Autodesk Inventor part; units mm, degrees
ref_plane "Work Plane1" through (0, 0, 6.25) normal (0, 0, 1) x (1, 0, 0)
ref_plane "YZ Plane" through (0, 0, 0) normal (1, 0, 0) x (0, 1, 0)
ref_plane "XZ Plane" through (0, 0, 0) normal (0, 1, 0) x (-1, 0, 0)
sketch "Sketch1" plane through (0, 0, 0) normal (0, 1, 0) x (-1, 0, 0)
  line L0 (0, -8.8201) -> (0, 9.1707)
  line L1 (0, -6.25) -> (0, 6.25)
  line L2 (0, -6.25) -> (1.5, -6.25)
  line L3 (1.5, -6.25) -> (1.5, 3.75)
  line L4 (1.5, 3.75) -> (2.75, 3.75)
  line L5 (2.75, 3.75) -> (2.75, 4.75)
  arc A0 (2.75, 4.75) -> (0, 6.25) centre (0, 2.9792) ccw
  line L6 (3.5295, 0) -> (-0.5882, 0)
  point P0 (0, 0)
  dimension "d0" = 10
  dimension "d1" = 3
  dimension "d2" = 2.5
  dimension "d3" = 5.5
  dimension "d4" = 1
revolve "Revolution1" add sketch "Sketch1" angle 360 about axis through (0, 0, -10) along (0, 0, 1)
ref_plane "Work Plane1" through (0, 0, 6.25) normal (0, 0, 1) x (1, 0, 0)
sketch "Sketch2" plane through (0, 0, 6.25) normal (0, 0, 1) x (1, 0, 0)
  line L0 (-1.35, -0.35) -> (1.35, -0.35)
  line L1 (1.35, -0.35) -> (1.35, 0.35)
  line L2 (1.35, 0.35) -> (-1.35, 0.35)
  line L3 (-1.35, 0.35) -> (-1.35, -0.35)
  line L4 (-1.35, -0.35) -> (1.35, 0.35) construction
  line L5 (1.35, -0.35) -> (-1.35, 0.35) construction
  line L6 (0.35, -1.35) -> (-0.35, -1.35)
  line L7 (-0.35, -1.35) -> (-0.35, 1.35)
  line L8 (-0.35, 1.35) -> (0.35, 1.35)
  line L9 (0.35, 1.35) -> (0.35, -1.35)
  line L10 (0.35, -1.35) -> (-0.35, 1.35) construction
  line L11 (-0.35, -1.35) -> (0.35, 1.35) construction
  point P0 (0, 0)
  dimension "d6" = 2.7
  dimension "d7" = 0.7
extrude "Extrusion1" cut sketch "Sketch2" against normal blind 1
thread "Thread1"
properties part number "empty"
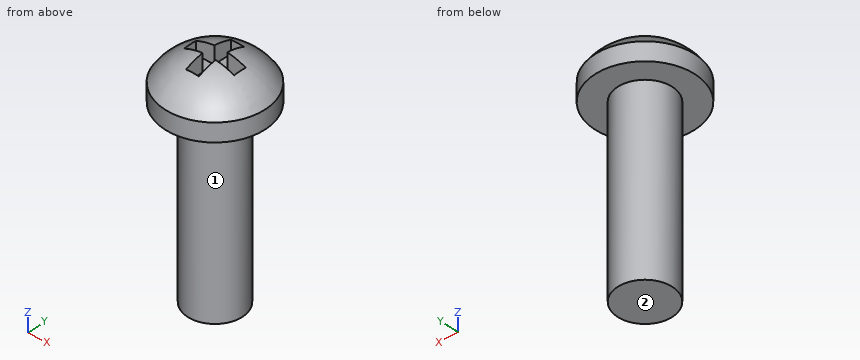
Design review of the part built by this model. Coordinates are the model's own, in mm. Face numbers are marked on the shaded views. A direction names the side the tool comes from. Round coordinates to 2 decimals unless told otherwise and drop trailing zeros. Loops run counter-clockwise (first coordinate to the right, second up) from the corner with the lowest first, then second, coordinate; pieces in that order, holes last. Notation, with made-up numbers: (16.5, -14.75) - (41.5, -14.75) arc R24 ccw to (41.5, 6.25) - close; hole circle Ø5 at (59, -35.5). An arc over 180 degrees is marked (long way). One line per item, written item: value. Start each with the question number.
1) Consider section A-A on z = -1.75. Give the boundary of the cut face in (x, y).
2) Consider section B-B on z = 4.5. Give the boundary of the cut face in (x, y), then the cut area to 3 significant figures.
3) Insertion check: pin 1 Ø3 at (x, y) = (-2, 1) entering from +Z; pin 2 Ø1.1 at (x, z) = (1, 5.5) entering from -Y; pin 3 Ø0.6 at (x, z) = (0, 5.5) entering from +Y. Each pin has a flat end and moves straight along its axis. Give the tip position at first contact, or say it passes through.
4) For the marked faces 1 and 2, list the 3-axis set-ups (+Z, -Z, +X, -X, +Y, -Y) from which the entire face can be reached by the end or side of a thin tool; tool diameter is ignored.
5) To check wall thickness, follow L1, parallel to Y at x = -0.05, z = -1.75; L2, parallel to Z at x = 0.3, y = 1; L3, parallel to Z at x = -1.6, y = 0.1. State the ranges of each line that lie inside material, in increasing order. Write a range as from..to.
Reported:
1. outline: circle Ø3 at (0, 0)
2. outline: circle Ø5.5 at (0, 0)
2. area: 23.8 mm^2
3. pin 1: stops at z = 6.17
3. pin 2: stops at y = -2.45
3. pin 3: stops at y = 2.4
4. face 1: -Z
4. face 2: -Z, +X, -X, +Y, -Y
5. L1: y = -1.5..1.5
5. L2: z = -6.25..5.25
5. L3: z = 3.75..5.83
